Design review of the part built by this model. Coordinates are the model's own, in mm. Give positions to 0.01 mm unless a question says otherwise; leave off trailing zeros. Write each loop counter-clockwise with the first axis right and the second up, starting at its lowest first coordinate (ties: lowest second). Pieces come first, ordered by that corner, then holes. Notation, with made-up numbers: (6.25, 78.5) -> (30.25, 78.5) arc R25 ccw to (30.25, 102.5) -> close; hole circle Ø5 at (-26, 23.5). An arc over 180 degrees is marked (long way). Answer as a JSON object with one key per item and string values.
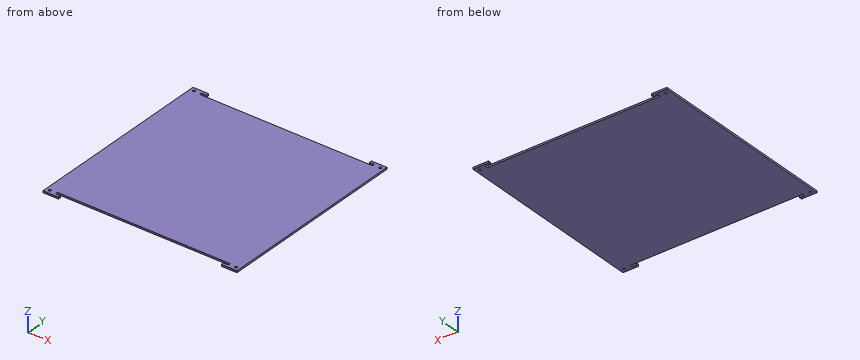
```python
from build123d import *

# Parameters (mm, degrees)
SKETCH_R      = 3.9751
EXTRUDE_DEPTH = 5.9944


with BuildPart() as part:
    # Sketch → Extrude (new body)
    with BuildSketch(Plane.XY):
        with BuildLine():
            Line((0, 0), (0, -635))
            Line((0, -635), (50.8, -635))
            Line((50.8, -635), (50.8, -626.2751))
            Line((50.8, -626.2751), (38.1, -626.2751))
            ThreePointArc((38.1, -618.3249), (34.1249, -622.3), (38.1, -626.2751))
            Line((38.1, -618.3249), (596.9, -618.3249))
            ThreePointArc((596.9, -626.2751), (600.8751, -622.3), (596.9, -618.3249))
            Line((584.2, -626.2751), (596.9, -626.2751))
            Line((584.2, -635), (584.2, -626.2751))
            Line((635, -635), (584.2, -635))
            Line((635, 0), (635, -635))
            Line((584.2, 0), (635, 0))
            Line((584.2, -8.7249), (584.2, 0))
            Line((584.2, -8.7249), (596.9, -8.7249))
            ThreePointArc((596.9, -16.6751), (600.8751, -12.7), (596.9, -8.7249))
            Line((38.1, -16.6751), (596.9, -16.6751))
            ThreePointArc((38.1, -8.7249), (34.1249, -12.7), (38.1, -16.6751))
            Line((50.8, -8.7249), (38.1, -8.7249))
            Line((50.8, 0), (50.8, -8.7249))
            Line((0, 0), (50.8, 0))
        make_face()
        with Locations((12.7, -12.7)):
            Circle(SKETCH_R, mode=Mode.SUBTRACT)
        with Locations((12.7, -622.3)):
            Circle(SKETCH_R, mode=Mode.SUBTRACT)
        with Locations((622.3, -12.7)):
            Circle(SKETCH_R, mode=Mode.SUBTRACT)
        with Locations((622.3, -622.3)):
            Circle(SKETCH_R, mode=Mode.SUBTRACT)
    extrude(amount=EXTRUDE_DEPTH)


solid = part.part
```
(1) For line 1 along Y through (x, z) = (622.3, 2.4); line 2 along X through (y, z) = (-622.3, 2.35); line 3 along Y through (x, z) = (550, 4.4), list the stretches that pass through material, from the lowest coordinate up.
Here are the results:
{"line 1": "y = -635 to -626.28, -618.32 to -16.68, -8.72 to 0", "line 2": "x = 0 to 8.72, 16.68 to 34.12, 600.88 to 618.32, 626.28 to 635", "line 3": "y = -618.32 to -16.68"}
(2) We need section A-A, the plane z = 3.25. State the section outline as (x, y) points, then the cut area to 3 significant figures.
Here are the results:
{"outline": "(0, -635) -> (50.8, -635) -> (50.8, -626.28) -> (38.1, -626.28) arc R3.98 cw to (38.1, -618.32) -> (596.9, -618.32) arc R3.98 cw to (596.9, -626.28) -> (584.2, -626.28) -> (584.2, -635) -> (635, -635) -> (635, 0) -> (584.2, 0) -> (584.2, -8.72) -> (596.9, -8.72) arc R3.98 cw to (596.9, -16.68) -> (38.1, -16.68) arc R3.98 cw to (38.1, -8.72) -> (50.8, -8.72) -> (50.8, 0) -> (0, 0) -> close; hole circle Ø7.95 at (12.7, -622.3); hole circle Ø7.95 at (12.7, -12.7); hole circle Ø7.95 at (622.3, -622.3); hole circle Ø7.95 at (622.3, -12.7)", "area": "385,000 mm²"}
(3) Clearance check with flat-ended pins moving along their axes: pin 1 (3 mm diameter, centred on x = 333, z = 1.5, fed in from +Y); pin 2 (1.8 mm diameter, centred on x = 325, z = 1.5, fed in from -Y). State where each tip first meets the part, or that it passes through.
Here are the results:
{"pin 1": "stops at y = -16.68", "pin 2": "stops at y = -618.32"}
(4) We need section B-B, the plane x = 235.5. State the section outline as (y, z) points.
Here are the results:
{"outline": "(-618.32, 0) -> (-16.68, 0) -> (-16.68, 5.99) -> (-618.32, 5.99) -> close"}
